```python
from build123d import *

# Parameters (mm, degrees)
SKETCH1_R                = 38.1
SKETCH1_R_2              = 31.75
BOSS_EXTRUDE1_DEPTH      = 55.372
BOSS_EXTRUDE2_REACH      = 115.998
BOSS_EXTRUDE2_END_RADIUS = 38.1
SKETCH2_W                = 3.048
SKETCH2_H                = 55.372
CIRPATTERN1_COUNT        = 8


with BuildPart() as part:
    # Sketch1 → Boss-Extrude1 (new body)
    with BuildSketch(Plane(origin=(0, 0, 0), x_dir=(1, 0, 0), z_dir=(0, 1, 0))):
        with Locations(Location((0, 0, 0), (0, 0, 270))):
            Circle(SKETCH1_R)
        with Locations(Location((0, 0, 0), (0, 0, 270))):
            Circle(SKETCH1_R_2, mode=Mode.SUBTRACT)
    extrude(amount=BOSS_EXTRUDE1_DEPTH)

    # Boss-Extrude2: up to this cylinder (the profile starts outside it)
    boss_extrude2_end = Plane(origin=(0, 27.686, 0), z_dir=(0, -1, 0)) * Cylinder(BOSS_EXTRUDE2_END_RADIUS, 309.196, mode=Mode.PRIVATE)
    # Sketch2 → Boss-Extrude2 (add, up to the surface)
    with BuildSketch(Plane.XY.offset(53.975), mode=Mode.PRIVATE) as boss_extrude2_sk1:
        with Locations((0, 27.686)):
            Rectangle(SKETCH2_W, SKETCH2_H)
    boss_extrude2_tool1 = extrude(boss_extrude2_sk1.sketch, amount=-BOSS_EXTRUDE2_REACH, mode=Mode.PRIVATE) - boss_extrude2_end
    boss_extrude2 = boss_extrude2_tool1.solids().sort_by_distance((0, 27.686, 53.975))[0]
    add(boss_extrude2)

    # CirPattern1: Boss-Extrude2 ×8 about axis
    cirpattern1_axis = Axis((0, 0, 0), (0, 1, 0))
    for i in range(1, CIRPATTERN1_COUNT):
        add(boss_extrude2.rotate(cirpattern1_axis, i * 360 / CIRPATTERN1_COUNT))


solid = part.part
```
Could you check a few things on this model? Use its own coordinates, in mm. A direction names the side the tool comes from. Round coordinates to 2 decimals unless told otherwise and drop trailing zeros. Write each loop counter-clockwise with the first axis right and the second up, starting at its lowest first coordinate (ties: lowest second). Pieces come first, ordered by that corner, then holes. Notation, with made-up numbers: M 55,-22.75 L 65,-22.75 A29 ccw 65,4.25 Z; hole C 17.25,40 d1. An arc over 180 degrees is marked long. Answer in a Markdown table with one row per item. Add a question column.
Q1. Will these pins go through, and if not, where does the flat tip stop? pin 1 Ø17.5 at (x, y) = (-49, 29) entering from +Z; pin 2 Ø17.5 at (x, y) = (-43.5, 29) entering from -Z; pin 3 Ø12.5 at (y, z) = (28.5, 44) entering from -X; pin 4 Ø10 at (x, z) = (37.5, -4) entering from -Y.
Q2. Imagine slicing it at D-D (z = 41.5). Please give me the cut outline in (x, y), then the cut area to 3 significant figures.
Q3. If I drill on line 1 (X direction, y = 18, z = 0) (3 decimals); line 2 (X direction, y = 30, z = 34); line 3 (X direction, y = 45.5, z = -17), over which ranges is the centre line in solid material (lowest first)? Write a range as from..to.
Q4. Imagine slicing it at B-B (x = 0). Please give me the cut outline in (y, z) (3 decimals), then the cut area to 3 significant figures.
Q5. Imagine slicing it at A-A (z = 0). Please give me the cut outline in (x, y) (3 decimals).
Q6. On a 3-axis mill with a long thin cutter (end or side, diameter ignored), from which of +Z, -Z, +X, -X, +Y, -Y can I reach the whole of each face in a straight line? I mean faces 1 (the flat face through (-33.699, 27.298, -31.544)), 2 (the flat face through (53.975, 28, 0)), 3 (the flat face through (-31.544, 27.298, 33.699)), 4 (the cylindrical face through (35.13, 27.3, 14.75)), 5 (the flat face through (31.544, 27.298, -33.699)). Say none if no direction works.
Q7. If we mould it in two halves opening along Z, with no side actions, what happens to faces 6 (the cylindrical face through (-30.995, 27.298, -6.883)), 7 (the flat face through (-1.524, 27, 46)), 8 (the cylindrical face through (14.41, 27.3, 35.27))? For each: +Z half, -Z half, draft (parallel to the pull), parting line (faces both ways), or undercut.
Values:
| question | item | result |
|---|---|---|
| 1 | pin 1 | z = 1.52 |
| 1 | pin 2 | z = -39.24 |
| 1 | pin 3 | x = -38.58 |
| 1 | pin 4 | y = 0 |
| 2 | outline | M -1.52,0 L 1.52,0 L 1.52,55.37 L -1.52,55.37 Z |
| 2 | area | 169 mm^2 |
| 3 | line 1 | -53.975..-31.75, 31.75..53.975 |
| 3 | line 2 | -36.16..-31.84, -17.19..17.19, 31.84..36.16 |
| 3 | line 3 | -34.1..-26.82, 26.82..34.1 |
| 4 | outline | M 0,-53.975 L 55.372,-53.975 L 55.372,-31.75 L 0,-31.75 Z; M 0,31.75 L 55.372,31.75 L 55.372,53.975 L 0,53.975 Z |
| 4 | area | 2,460 mm^2 |
| 5 | outline | M -53.975,0 L -31.75,0 L -31.75,55.372 L -53.975,55.372 Z; M 31.75,0 L 53.975,0 L 53.975,55.372 L 31.75,55.372 Z |
| 6 | face 1 | -X, +Y, -Y |
| 6 | face 2 | +Z, -Z, +X, +Y, -Y |
| 6 | face 3 | +Z, +Y, -Y |
| 6 | face 4 | +X, +Y, -Y |
| 6 | face 5 | -Z, +Y, -Y |
| 7 | face 6 | undercut |
| 7 | face 7 | draft |
| 7 | face 8 | +Z half |
